Source: three-view drawing plus pictorial views. Frame: mm from the lowest corner of the part. Give positions to 0.01 mm unless a question says otherwise; leave off trailing zeros. Loops run counter-clockwise (first coordinate to the right, second up) from the corner with the lowest first, then second, coordinate; pieces in that order, holes last. Notation, with made-up numbers: M 21.5,89.5 L 31.5,89.5 A19 ccw 31.5,107.5 Z; hole C 26,8 d9. An arc over 180 degrees is marked long. One line per item, written item: value. Start each with the question number.
(1) Section D-D on x = 1.8. Output: boundary loops of the cut face in (y, z).
(2) Pin query (flat end, axial travel): P1, Ø3, axis at x = 1.5, y = 14.5, coming from the -Z side; P2, Ø1, axis at x = 0.5, z = 1, coming from the -Y side. Return the tip coordinate at first contact, or that it passes through.
(3) Ray query, line 1 along Y through (x, z) = (3, 1.15); line 2 along Y through (x, z) = (4.2, 1.3); line 3 along Y through (x, z) = (5.3, 0.3). Return the intervals inside material, ascending. Write a range as from..to.
(4) Section B-B on x = 3. Output: boundary loops of the cut face in (y, z), plus the area to 3 significant figures.
(5) Section A-A on y = 16. Output: boundary loops of the cut face in (x, z), plus the area to 3 significant figures.
(6) Section C-C on z = 0.8. Output: boundary loops of the cut face in (x, y).
(7) Pull-direction query (X, two-part tool) for the marked faces 1, 2 and 3; classes: released by +X, released by -X, zero draft, split by the parting line, or undercut.
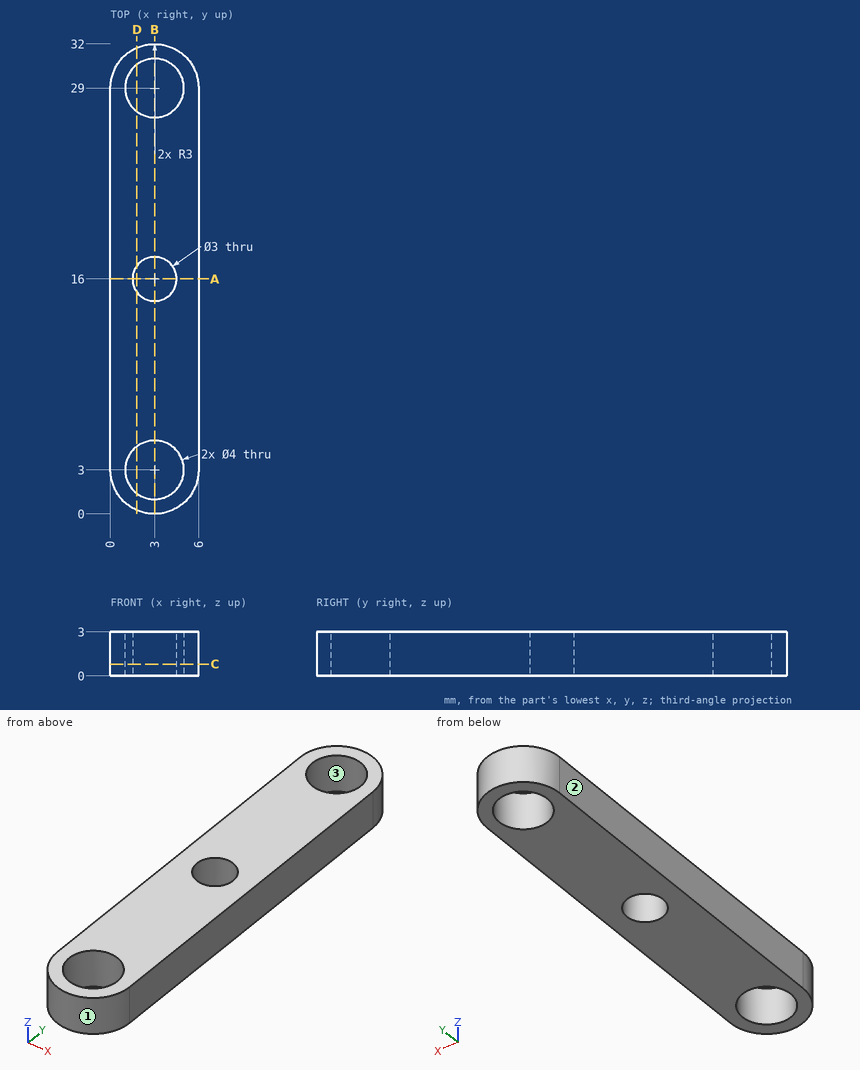
Output values:
1. outline: M 0.25,0 L 1.4,0 L 1.4,3 L 0.25,3 Z; M 4.6,0 L 15.1,0 L 15.1,3 L 4.6,3 Z; M 16.9,0 L 27.4,0 L 27.4,3 L 16.9,3 Z; M 30.6,0 L 31.75,0 L 31.75,3 L 30.6,3 Z
2. P1: stops at z = 0
2. P2: stops at y = 0.76
3. line 1: y = 0..1, 5..14.5, 17.5..27, 31..32
3. line 2: y = 0.25..1.4, 4.6..15.1, 16.9..27.4, 30.6..31.75
3. line 3: y = 1.07..30.93
4. outline: M 0,0 L 1,0 L 1,3 L 0,3 Z; M 5,0 L 14.5,0 L 14.5,3 L 5,3 Z; M 17.5,0 L 27,0 L 27,3 L 17.5,3 Z; M 31,0 L 32,0 L 32,3 L 31,3 Z
4. area: 63.0 mm²
5. outline: M 0,0 L 1.5,0 L 1.5,3 L 0,3 Z; M 4.5,0 L 6,0 L 6,3 L 4.5,3 Z
5. area: 9.00 mm²
6. outline: M 0,3 A3 ccw 6,3 L 6,29 A3 ccw 0,29 Z; hole C 3,3 d4; hole C 3,29 d4; hole C 3,16 d3
7. face 1: split by the parting line
7. face 2: released by -X
7. face 3: undercut
